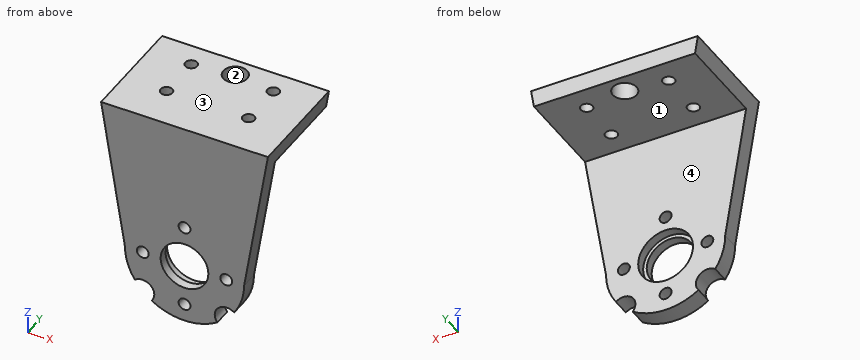
from build123d import *

# Parameters (mm, degrees)
BOSS_EXTRUDE1_DEPTH = 3
SKETCH2_R           = 4
CUT_EXTRUDE1_DEPTH  = 13
SKETCH4_R           = 1
CUT_EXTRUDE3_DEPTH  = 3
BOSS_EXTRUDE2_DEPTH = 15.5
SKETCH6_R           = 4.6
CUT_EXTRUDE4_DEPTH  = 1.5
SKETCH7_R           = 2
CUT_EXTRUDE5_DEPTH  = 10
SKETCH8_R           = 1
CUT_EXTRUDE6_DEPTH  = 10
SKETCH9_R           = 2
CUT_EXTRUDE7_DEPTH  = 10


with BuildPart() as part:
    # Sketch1 → Boss-Extrude1 (new body)
    with BuildSketch(Plane(origin=(0, 0, 0), x_dir=(1, 0, 0), z_dir=(0, 1, 0))):
        with BuildLine():
            Line((-10, 0), (-14, -25))
            Line((-14, -25), (14, -25))
            Line((14, -25), (10, 0))
            ThreePointArc((10, 0), (0, 10), (-10, 0))
        make_face()
    extrude(amount=BOSS_EXTRUDE1_DEPTH)

    # Sketch2 → Cut-Extrude1 (cut)
    with BuildSketch(Plane(origin=(0, 3, 0), x_dir=(1, 0, 0), z_dir=(0, 1, 0))):
        Circle(SKETCH2_R)
    extrude(amount=-CUT_EXTRUDE1_DEPTH, mode=Mode.SUBTRACT)

    # Sketch4 → Cut-Extrude3 (cut)
    with BuildSketch(Plane(origin=(0, 3, 0), x_dir=(1, 0, 0), z_dir=(0, 1, 0))):
        with Locations((0, -7)):
            Circle(SKETCH4_R)
        with Locations((-7, 0)):
            Circle(SKETCH4_R)
        with Locations((0, 7)):
            Circle(SKETCH4_R)
        with Locations((7, 0)):
            Circle(SKETCH4_R)
    extrude(amount=-CUT_EXTRUDE3_DEPTH, mode=Mode.SUBTRACT)

    # Sketch5 → Boss-Extrude2 (add)
    with BuildSketch(Plane(origin=(0, 3, 0), x_dir=(1, 0, 0), z_dir=(0, 1, 0))):
        Polygon((-13.52, -22), (13.52, -22), (14, -25), (-14, -25), align=None)
    extrude(amount=BOSS_EXTRUDE2_DEPTH)

    # Sketch6 → Cut-Extrude4 (cut)
    with BuildSketch(Plane(origin=(0, 3, 0), x_dir=(1, 0, 0), z_dir=(0, 1, 0))):
        Circle(SKETCH6_R)
    extrude(amount=-CUT_EXTRUDE4_DEPTH, mode=Mode.SUBTRACT)

    # Sketch7 → Cut-Extrude5 (cut)
    with BuildSketch(Plane(origin=(0, 3, 0), x_dir=(1, 0, 0), z_dir=(0, 1, 0))):
        with Locations((-7.071067812, 7.071067812)):
            Circle(SKETCH7_R)
        with Locations((7.071067812, 7.071067812)):
            Circle(SKETCH7_R)
    extrude(amount=-CUT_EXTRUDE5_DEPTH, mode=Mode.SUBTRACT)

    # Sketch8 → Cut-Extrude6 (cut)
    with BuildSketch(Plane(origin=(0, 0, 22), x_dir=(-1, 0, 0), z_dir=(0, 0, -1))):
        with Locations((6.885, 7)):
            Circle(SKETCH8_R)
        with Locations((-6.885, 7)):
            Circle(SKETCH8_R)
        with Locations((6.885, 14.5)):
            Circle(SKETCH8_R)
        with Locations((-6.885, 14.5)):
            Circle(SKETCH8_R)
    extrude(amount=-CUT_EXTRUDE6_DEPTH, mode=Mode.SUBTRACT)

    # Sketch9 → Cut-Extrude7 (cut)
    with BuildSketch(Plane(origin=(0, 0, 22), x_dir=(-1, 0, 0), z_dir=(0, 0, -1))):
        with Locations((0, 15.4)):
            Circle(SKETCH9_R)
    extrude(amount=-CUT_EXTRUDE7_DEPTH, mode=Mode.SUBTRACT)


solid = part.part
Source: CAD feature listing. Evaluate the final solid. Frame: model axes, mm. Face numbers are marked on the shaded views. A direction names the side the tool comes from. Round coordinates to 2 decimals unless told otherwise and drop trailing zeros. Loops run counter-clockwise (first coordinate to the right, second up) from the corner with the lowest first, then second, coordinate; pieces in that order, holes last. Notation, with made-up numbers: M 63.25,30 L 121.25,30 A31 ccw 121.25,69 Z; hole C 36.5,69.25 d4. An arc over 180 degrees is marked long. Answer as CSV lines item,"result".
Q1. Cut plane B-B (x = 0). Return the cut outline in (y, z).
Verdict:
outline,"M 0,-10 L 3,-10 L 3,-8 L 0,-8 Z; M 0,-6 L 3,-6 L 3,-4.6 L 1.5,-4.6 L 1.5,-4 L 0,-4 Z; M 0,4 L 1.5,4 L 1.5,4.6 L 3,4.6 L 3,6 L 0,6 Z; M 0,8 L 3,8 L 3,22 L 13.4,22 L 13.4,25 L 0,25 Z; M 17.4,22 L 18.5,22 L 18.5,25 L 17.4,25 Z"
Q2. Pull-direction query (X, two-part tool) for the marked faces 1 and 2; classes: +X half, -X half, draft (parallel to the pull), parting line (faces both ways), or undercut.
Verdict:
face 1,"draft"
face 2,"undercut"
Q3. Cut plane A-A (y = 7). Return the cut outline in (x, z) (3 decimals), plus the area to 3 significant figures.
Verdict:
outline,"M -14,25 L -13.52,22 L -7.885,22 L -7.885,25 Z; M -5.885,22 L 5.885,22 L 5.885,25 L -5.885,25 Z; M 7.885,22 L 13.52,22 L 14,25 L 7.885,25 Z"
area,"70.6 mm^2"
Q4. Line query: line 1 along X through (y, z) = (2.05, 0); line 2 along X through (y, z) = (1.1, 0); line 3 along Z through (x, y) = (-7, 1.05). Output: solid intervals per line, ascending.
Verdict:
line 1,"x = -10 to -8, -6 to -4.6, 4.6 to 6, 8 to 10"
line 2,"x = -10 to -8, -6 to -4, 4 to 6, 8 to 10"
line 3,"z = -5.07 to -1, 1 to 25"
Q5. Cut plane D-D (x = -11). Return the cut outline in (y, z), plus the area to 3 significant figures.
Verdict:
outline,"M 0,6.25 L 3,6.25 L 3,22 L 18.5,22 L 18.5,25 L 0,25 Z"
area,"103 mm^2"
Q6. Contact query for flat-ended pins moving along their axis: pin 1 (3 mm diameter, centred on x = 0, y = 15.4, fed in from +Z); pin 2 (3 mm diameter, centred on x = 0, z = -7, fed in from +Y); pin 3 (5 mm diameter, centred on x = 10, z = 5, fed in from -Y); pin 4 (8 mm diameter, centred on x = -4, y = 10.5, fed in from -Z). Output: stop coordinate, or through.
Verdict:
pin 1,"passes through"
pin 2,"stops at y = 3"
pin 3,"stops at y = 0"
pin 4,"stops at z = 22"
Q7. Reachability of the marked faces 3 and 4 from +Z, -Z, +X, -X, +Y, -Y: full face, straight path, thin tool, end or side. Return the list, or none.
Verdict:
face 3,"+Z, +X, -X, +Y, -Y"
face 4,"-Z, +X, -X, +Y"
Q8. Cut plane C-C (y = 14.5). Return the cut outline in (x, z) (3 decimals).
Verdict:
outline,"M -14,25 L -13.52,22 L -7.885,22 L -7.885,25 Z; M -5.885,22 L -1.786,22 L -1.786,25 L -5.885,25 Z; M 1.786,22 L 5.885,22 L 5.885,25 L 1.786,25 Z; M 7.885,22 L 13.52,22 L 14,25 L 7.885,25 Z"
